For this review, take the finished solid that the model builds, in its own axes (mm). A direction names the side the tool comes from. Coordinates: 2 decimals unless noted, no trailing zeros. Loops run counter-clockwise (first coordinate to the right, second up) from the corner with the lowest first, then second, coordinate; pieces in that order, holes last. Notation, with made-up numbers: M 6.25,70 L 48.25,70 A10 ccw 48.25,86 Z; hole C -39,4 d9. An arc over 180 degrees is marked long. Answer as a JSON object with one key per item and string values. Group by question number.
Item 1: Add section D-D (y = -3). Count the separate pieces of the cut face and the enclosed holes in it, then the cut area to 3 significant figures.
Item 2: Add section B-B (z = 22.25). State the section outline as (x, y) points, then the cut area to 3 significant figures.
Item 3: Insertion check: pin 1 (6 mm diameter, centred on x = 33, y = 1, fed in from +Z); pin 2 (1 mm diameter, centred on x = -58.5, z = 25, fed in from +Y); pin 3 (0.5 mm diameter, centred on x = 58.5, z = 20, fed in from -Y). Each pin has a flat end and moves straight along its axis. Give the tip position at first contact, or say it passes through.
Item 4: Mouldability with a two-part tool opening along Y and no side actions: class faces 3 (the face through (58, 8, 4)), 4 (the face through (-59, 0, 26)), 5 (the face through (-65, 0, 2)) as +Y half, -Y half, draft (parallel to the pull), parting line (faces both ways), or undercut.
Item 5: Add section A-A (x = 50.5). State the section outline as (y, z) points.
Item 6: Add section C-C (x = -25.5). State the section outline as (y, z) points.
Item 7: Wall thickness on L1, parallel to Y at x = 50.5, z = 1.3; L2, parallel to Y at x = -30, z = 4; L3, parallel to Z at x = 49.5, y = -2.25: over which ranges is each line inside the solid? List them lowest first. Write a range as from..to.
Item 8: Tool access review of faces 1 (the face through (-59, 8, 4)), 2 (the face through (-1, -12.5, 2)): name each direction out of +Z, -Z, +X, -X, +Y, -Y from which nothing blocks a thin tool from reaching the whole face with its end or side.
from build123d import *

# Parameters (mm, degrees)
F0_W      = 130
F0_H      = 25
F1_DEPTH  = 5
F2_T      = -2.5
F3_W      = 4
F3_H      = 16
F4_DEPTH  = 25
F6_DEPTH  = 125.501
F7_R      = 1.5
F8_R      = 1.5
F9_R      = 1.75
F10_DEPTH = 2.501


with BuildPart() as f1:
    # F0 (on Top) → F1 (new body)
    with BuildSketch(Plane.XY):
        Rectangle(F0_W, F0_H)
    extrude(amount=F1_DEPTH)

    # F2
    f2_openings = [f1.faces().sort_by_distance(p)[0] for p in [
        (0, 0, 5),
    ]]
    offset(amount=F2_T, openings=f2_openings)

    # F3 (on face) → F4 (join)
    with BuildSketch(Plane.XY.offset(2.5)):
        with Locations((-58.5, 0)):
            Rectangle(F3_W, F3_H)
        with Locations((58.5, 0)):
            Rectangle(F3_W, F3_H)
    extrude(amount=F4_DEPTH)

    # F5 (on face) → F6 (cut, through all)
    with BuildSketch(Plane(origin=(-60.5, 0, 0), x_dir=(0, -1, 0), z_dir=(-1, 0, 0))):
        Polygon((0, 24), (0, 27.5), (-8, 27.5), (-8, 5.5), (4.5, 10.5), (4.5, 24), align=None)
    extrude(amount=-F6_DEPTH, mode=Mode.SUBTRACT)

    # F7
    f7_edges = [f1.edges().sort_by_distance(p)[0] for p in [
        (-60.5, -2.25, 24),
        (-60.5, -4, 27.5),
        (-56.5, -4, 27.5),
        (-56.5, -2.25, 24),
        (-60.5, -4.5, 17.25),
        (-56.5, -4.5, 17.25),
        (-60.5, -8, 15),
        (-56.5, -8, 15),
        (-60.5, 1.75, 8),
        (-56.5, 1.75, 8),
    ]]
    fillet(f7_edges, radius=F7_R)

    # F8
    f8_edges = [f1.edges().sort_by_distance(p)[0] for p in [
        (60.5, -4, 27.5),
        (56.5, -4, 27.5),
        (60.5, -2.25, 24),
        (60.5, -4.5, 17.25),
        (60.5, -8, 15),
        (60.5, 1.75, 8),
        (56.5, -8, 15),
        (56.5, -4.5, 17.25),
        (56.5, -2.25, 24),
        (56.5, 1.75, 8),
    ]]
    fillet(f8_edges, radius=F8_R)

    # F9 (on face) → F10 (cut, through all)
    with BuildSketch(Plane.XY.offset(2.5)):
        with Locations((-50.5, 0)):
            Circle(F9_R)
        with Locations((50.5, 0)):
            Circle(F9_R)
    extrude(amount=-F10_DEPTH, mode=Mode.SUBTRACT)


solid = f1.part
From the geometry:
{
 "1": {"separate pieces": "3", "enclosed holes": "0", "area": "419 mm²"},
 "2": {"outline": "M -60.5,-6.5 A1.5 ccw -59,-8 L -58,-8 A1.5 ccw -56.5,-6.5 L -56.5,-6 A1.5 ccw -58,-4.5 L -59,-4.5 A1.5 ccw -60.5,-6 Z; M 56.5,-6.5 A1.5 ccw 58,-8 L 59,-8 A1.5 ccw 60.5,-6.5 L 60.5,-6 A1.5 ccw 59,-4.5 L 58,-4.5 A1.5 ccw 56.5,-6 Z", "area": "24.1 mm²"},
 "3": {"pin 1": "stops at z = 2.5", "pin 2": "stops at y = 0", "pin 3": "stops at y = -8"},
 "4": {"face 3": "undercut", "face 4": "+Y half", "face 5": "draft"},
 "5": {"outline": "M -12.5,0 L -1.75,0 L -1.75,2.5 L -10,2.5 L -10,5 L -12.5,5 Z; M 1.75,0 L 12.5,0 L 12.5,5 L 10,5 L 10,2.5 L 1.75,2.5 Z"},
 "6": {"outline": "M -12.5,0 L 12.5,0 L 12.5,5 L 10,5 L 10,2.5 L -10,2.5 L -10,5 L -12.5,5 Z"},
 "7": {"L1": "y = -12.5..-1.75, 1.75..12.5", "L2": "y = -12.5..-10, 10..12.5", "L3": "z = 0..2.5"},
 "8": {"face 1": "+Z", "face 2": "+Z, -Z, +X, -X, -Y"}
}
